Input: dimensioned drawing with shaded views. Units: mm. Origin: part minimum x, y, z. A direction names the side the tool comes from. Round coordinates to 2 decimals unless told otherwise and drop trailing zeros. Order: outer loops, then holes, each group sorted by start corner. A loop starts at its lowest first (then second) coordinate and runs counter-clockwise, first axis right, second up. Notation, with made-up numbers: (63, 15.25) - (67, 15.25) arc R25 cw to (67, 52.25) - close; hole circle Ø6 at (5.25, 17). An arc over 180 degrees is marked (long way). Return JSON: item names as keys, results as strings. Group by question number.
1) Section D-D, the plane x = 5. Return loops of the section in (y, z).
2) Section B-B, the plane z = 2. Return loops of the section in (x, y) (1 decimal).
3) Contact query for flat-ended pins moving along their axis: P1, Ø1.9, axis at y = 4, z = 4.5, coming from the -X side; P2, Ø1.5, axis at y = 3.5, z = 0.5, coming from the -X side. Output: stop coordinate, or through.
4) Section A-A, the plane x = 3.75. Return loops of the section in (y, z).
5) Ray query, line 1 (Y direction, x = 5.5, z = 2.25); line 2 (X direction, y = 5.5, z = 5.25) (1 decimal); line 3 (X direction, y = 2.25, z = 1.75) (1 decimal). Return the intervals inside material, ascending. Write a range as from..to.
6) Mould query, pull axis X, two halves, no side actions, for the marked faces 1, 2 and 3. Classes: pulls with the +X half, pulls with the -X half, needs draft (parallel to the pull), parting line crosses it, or undercut.
7) Access query for the marked faces 4, 5 and 6. Directions: +Z, -Z, +X, -X, +Y, -Y. A direction counts if a zero-diameter tool reaches every point of the face in a straight line with its end or side. Return the directions, or none.
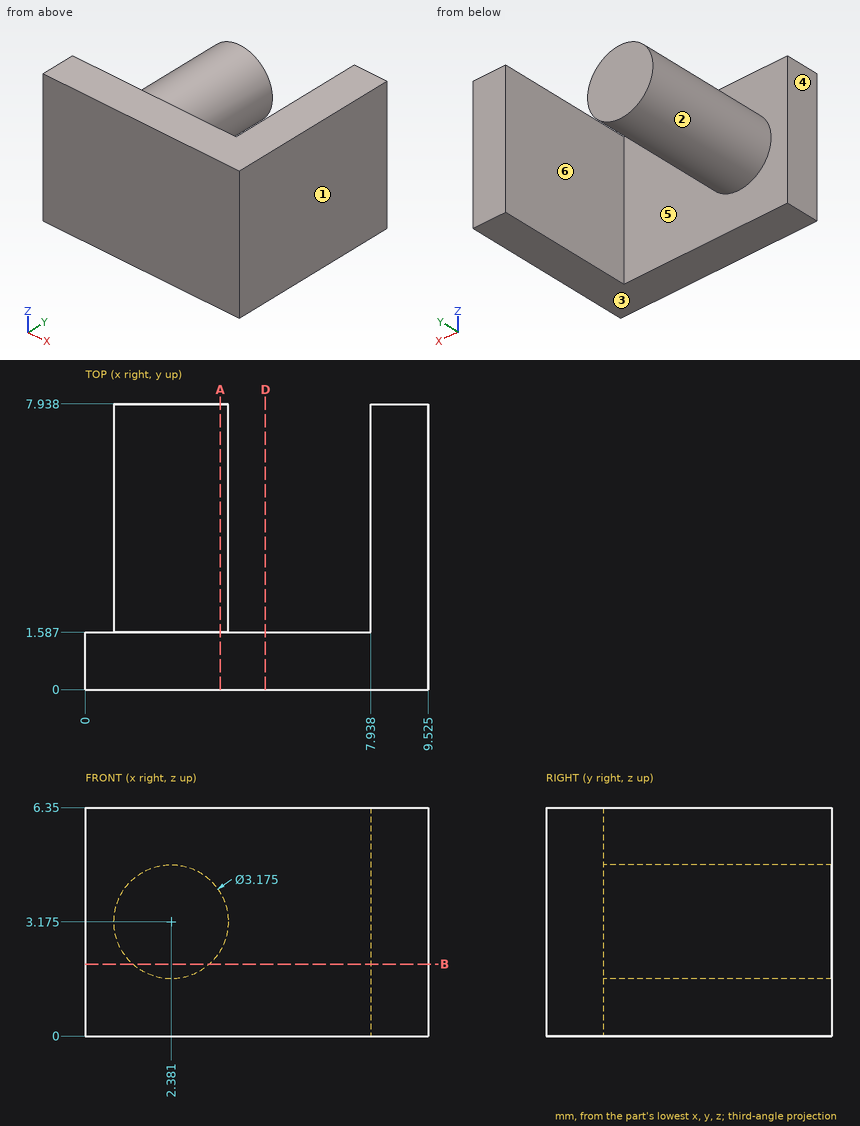
Geometry check:
{
 "1": {"outline": "(0, 0) - (1.59, 0) - (1.59, 6.35) - (0, 6.35) - close"},
 "2": {"outline": "(0, 0) - (9.5, 0) - (9.5, 7.9) - (7.9, 7.9) - (7.9, 1.6) - (3.4, 1.6) - (3.4, 7.9) - (1.3, 7.9) - (1.3, 1.6) - (0, 1.6) - close"},
 "3": {"P1": "x = 0.84", "P2": "x = 7.94"},
 "4": {"outline": "(0, 0) - (1.59, 0) - (1.59, 2.37) - (7.94, 2.37) - (7.94, 3.98) - (1.59, 3.98) - (1.59, 6.35) - (0, 6.35) - close"},
 "5": {"line 1": "0..1.59", "line 2": "7.9..9.5", "line 3": "1.7..3.1, 7.9..9.5"},
 "6": {"face 1": "pulls with the +X half", "face 2": "undercut", "face 3": "needs draft"},
 "7": {"face 4": "+Z, -Z, -X, +Y, -Y", "face 5": "+Y", "face 6": "+Z, -Z, +Y"}
}
